from build123d import *

# Parameters (mm, degrees)
SKETCH1_R           = 12.7
BOSS_EXTRUDE1_DEPTH = 12.7
BOSS_EXTRUDE2_DEPTH = 8.89
CUT_EXTRUDE1_REACH  = 36.662
SKETCH4_R           = 0.6
SKETCH5_R           = 6.3754
CUT_EXTRUDE2_DEPTH  = 11.83132


with BuildPart() as part:
    # Sketch1 → Boss-Extrude1 (new body)
    with BuildSketch(Plane(origin=(0, 0, 0), x_dir=(1, 0, 0), z_dir=(0, 1, 0))):
        with Locations(Location((0, 0, 0), (0, 0, 270))):
            Circle(SKETCH1_R)
    extrude(amount=BOSS_EXTRUDE1_DEPTH)

    # Sketch2 → Boss-Extrude2 (add)
    with BuildSketch(Plane(origin=(0, 0, 0), x_dir=(-1, 0, 0), z_dir=(0, -1, 0))):
        Polygon((-11.29479914, 9.353119572), (-13.747438724, -5.105023199), (-2.452639584, -14.458142772), (11.29479914, -9.353119572), (13.747438724, 5.105023199), (2.452639584, 14.458142772), align=None)
    extrude(amount=BOSS_EXTRUDE2_DEPTH)

    # Sketch3 → Revolve1 (revolve)
    with BuildSketch(Plane.XY, mode=Mode.PRIVATE) as revolve1_sk:
        Polygon((-1, -15.64499815), (-12.7, -8.89), (0, -8.89), (0, -15.64499815), align=None)
    revolve(revolve1_sk.sketch.rotate(Axis((0, -8.89, 0), (0, -1, 0)), 110.372156134), axis=Axis((0, -8.89, 0), (0, -1, 0)))

    # Sketch4 → Cut-Extrude1 (cut, up to next)
    with BuildSketch(Plane.XZ.offset(15.64499815), mode=Mode.PRIVATE) as cut_extrude1_sk1:
        with Locations(Location((0, 0, 0), (0, 0, 270))):
            Circle(SKETCH4_R)
    cut_extrude1_tool1 = extrude(cut_extrude1_sk1.sketch, amount=-CUT_EXTRUDE1_REACH, mode=Mode.PRIVATE) & part.part
    add(cut_extrude1_tool1.solids().sort_by_distance((0, -15.644998, 0))[0], mode=Mode.SUBTRACT)

    # Sketch5 → Cut-Extrude2 (cut)
    with BuildSketch(Plane(origin=(0, 12.7, 0), x_dir=(1, 0, 0), z_dir=(0, 1, 0))):
        with Locations(Location((0, 0, 0), (0, 0, 270))):
            Circle(SKETCH5_R)
    extrude(amount=-CUT_EXTRUDE2_DEPTH, mode=Mode.SUBTRACT)

    # Sketch6 → Cut-Revolve1 (revolve, cut)
    with BuildSketch(Plane.XY, mode=Mode.PRIVATE) as cut_revolve1_sk:
        Polygon((0, 0.86868), (6.3754, 0.86868), (0, -16.64758754), align=None)
    revolve(cut_revolve1_sk.sketch.rotate(Axis((0, 0.86868, 0), (0, -1, 0)), 270), axis=Axis((0, 0.86868, 0), (0, -1, 0)), mode=Mode.SUBTRACT)


solid = part.part
The listing builds one solid part. Answer for the finished solid, in the listing's coordinates (mm). A direction names the side the tool comes from. Coordinates: 2 decimals unless noted, no trailing zeros. Loops run counter-clockwise (first coordinate to the right, second up) from the corner with the lowest first, then second, coordinate; pieces in that order, holes last. Notation, with made-up numbers: (44.5, 6) -> (67.5, 6) arc R21 cw to (67.5, 22) -> close; hole circle Ø3 at (50.5, -22.75). An arc over 180 degrees is marked (long way). Answer in a Markdown table with one row per item. Add a question column.
1. Flat-ended cylindrical pins translate along their axes: P1, Ø5, axis at x = 4, z = 12, coming from the -Y side; P2, Ø2, axis at y = 6, z = 5.5, coming from the +X side; P3, Ø2.5, axis at x = -8, z = 7.5, coming from the -Y side. Find the tip coordinate at first contact, or state that the pin passes through.
2. For faces 5 (the cylindrical face through (-7.7, 6.3, -10.1)), 6 (the flat face through (-10.3, 0, 8.1)), 7 (the flat face through (-10.3, -8.89, 8.1)), determine the directions among +Z, -Z, +X, -X, +Y, -Y from which every point of the face is accessible in a straight line to the end or side of a thin tool.
3. The part is cut by section B-B, the plane y = 8. Write down the section's boundary in (x, z), then the cut area to 3 significant figures.
4. Consider line 1 (X direction, y = 9.5, z = 0); line 2 (X direction, y = -7.5, z = 5.5). Determine where each line is inside the solid, lowest interval first. Write a range as [from, to].
5. The part is cut by section A-A, the plane z = 0. Write down the section's boundary in (x, y) (3 decimals), then the cut area to 3 significant figures.
6. Determine the mould class of faces 1 (the flat face through (8.2, -4.4, 9.7)), 2 (the cylindrical face through (-2.44, 6.87, 5.89)), 3 (the flat face through (-12, -8.89, -5)), 4 (the flat face through (-8.2, -4.4, -9.7)) for opening direction X: +X half, -X half, draft (parallel to the pull), parting line (faces both ways), or undercut.
Answer below:
| question | item | result |
|---|---|---|
| 1 | P1 | y = -10.36 |
| 1 | P2 | x = 11.88 |
| 1 | P3 | y = -10.61 |
| 2 | face 5 | +Y |
| 2 | face 6 | +Z, -X, +Y |
| 2 | face 7 | +Z, -X, -Y |
| 3 | outline | circle Ø25.4 at (0, 0); hole circle Ø12.75 at (0, 0) |
| 3 | area | 379 mm2 |
| 4 | line 1 | [-12.7, -6.38], [6.38, 12.7] |
| 4 | line 2 | [-11.95, 13.27] |
| 5 | outline | (-12.881, -8.89) -> (-12.7, -8.89) -> (-1, -15.645) -> (-0.6, -15.645) -> (-0.6, -14.999) -> (-6.375, 0.869) -> (-6.375, 12.7) -> (-12.7, 12.7) -> (-12.7, 0) -> (-12.881, 0) -> close; (0.6, -15.645) -> (1, -15.645) -> (12.7, -8.89) -> (12.881, -8.89) -> (12.881, 0) -> (12.7, 0) -> (12.7, 12.7) -> (6.375, 12.7) -> (6.375, 0.869) -> (0.6, -14.999) -> close |
| 5 | area | 382 mm2 |
| 6 | face 1 | +X half |
| 6 | face 2 | undercut |
| 6 | face 3 | draft |
| 6 | face 4 | -X half |
